from build123d import *

# Parameters (mm, degrees)
BOSS_EXTRUDE1_DEPTH = 1.2


with BuildPart() as part:
    # Sketch1 → Boss-Extrude1 (new body)
    with BuildSketch(Plane(origin=(0, 0, 0), x_dir=(1, 0, 0), z_dir=(0, 1, 0))):
        with BuildLine():
            Line((-52.420457213, 58.5), (-52.420457213, 71.946194901))
            Line((-52.420457213, 71.946194901), (-60.488236819, 80.830210159))
            Line((-60.488236819, 80.830210159), (-65.373616564, 99.749725089))
            ThreePointArc((-65.373616564, 99.749725089), (-65.730427555, 101.60979478), (-65.85, 103.5))
            Line((-65.85, 103.5), (-124.130457213, 103.5))
            Line((-124.130457213, 103.5), (-124.130457213, -71.95))
            Line((-124.130457213, -71.95), (-112.891350531, -81.0301662))
            Line((-112.891350531, -81.0301662), (-108.397048281, -103.5))
            Line((-108.397048281, -103.5), (-52.420457213, -103.5))
            Line((-52.420457213, -103.5), (-52.420457213, -58.5))
            Line((-52.420457213, -58.5), (-50.420457213, -58.5))
            Line((-50.420457213, -58.5), (-50.420457213, -145.21))
            ThreePointArc((-50.420457213, -145.21), (-48.955991119, -148.745533906), (-45.420457213, -150.21))
            Line((-45.420457213, -150.21), (42.279542787, -150.21))
            ThreePointArc((42.279542787, -150.21), (45.815076693, -148.745533906), (47.279542787, -145.21))
            Line((47.279542787, -145.21), (47.279542787, -58.5))
            Line((47.279542787, -58.5), (49.279542787, -58.5))
            Line((49.279542787, -58.5), (49.279542787, -103.5))
            Line((49.279542787, -103.5), (105.256133855, -103.5))
            Line((105.256133855, -103.5), (109.750436105, -81.0301662))
            Line((109.750436105, -81.0301662), (120.989542787, -71.95))
            Line((120.989542787, -71.95), (120.989542787, -58.5))
            Line((120.989542787, -58.5), (242.489542787, -58.5))
            Line((242.489542787, -58.5), (242.489542787, 58.5))
            Line((242.489542787, 58.5), (217.489542787, 58.5))
            Line((217.489542787, 58.5), (217.489542787, 145.21))
            ThreePointArc((217.489542787, 145.21), (216.025076693, 148.745533906), (212.489542787, 150.21))
            Line((212.489542787, 150.21), (125.989542787, 150.21))
            ThreePointArc((125.989542787, 150.21), (122.454008881, 148.745533906), (120.989542787, 145.21))
            Line((120.989542787, 145.21), (120.989542787, 58.5))
            Line((120.989542787, 58.5), (119.489542787, 58.5))
            Line((119.489542787, 58.5), (119.489542787, 103.5))
            Line((119.489542787, 103.5), (62.709085574, 103.5))
            ThreePointArc((62.709085574, 103.5), (62.589513129, 101.60979478), (62.232702138, 99.749725089))
            Line((62.232702138, 99.749725089), (57.347322393, 80.830210159))
            Line((57.347322393, 80.830210159), (49.279542787, 71.946194901))
            Line((49.279542787, 71.946194901), (49.279542787, 58.5))
            Line((49.279542787, 58.5), (8.429542787, 58.5))
            ThreePointArc((8.429542787, 58.5), (-1.570457213, 48.5), (-11.570457213, 58.5))
            Line((-11.570457213, 58.5), (-52.420457213, 58.5))
        make_face()
    extrude(amount=BOSS_EXTRUDE1_DEPTH)


solid = part.part
Build history of the part. All positions in model axes, mm. A direction names the side the tool comes from. Round coordinates to 2 decimals unless told otherwise and drop trailing zeros. Loops run counter-clockwise (first coordinate to the right, second up) from the corner with the lowest first, then second, coordinate; pieces in that order, holes last. Notation, with made-up numbers: (-15.75, 67) -> (10.25, 67) arc R32 cw to (10.25, 93) -> close; hole circle Ø5 at (82.5, 86.25). An arc over 180 degrees is marked (long way). Answer in a Markdown table with one row per item.
Item 1: Saw through at A-A (z = 96). Write the cut outline in (x, y).
Answers below:
| item | result |
|---|---|
| outline | (-109.9, 0) -> (-52.42, 0) -> (-52.42, 1.2) -> (-109.9, 1.2) -> close; (-50.42, 0) -> (47.28, 0) -> (47.28, 1.2) -> (-50.42, 1.2) -> close; (49.28, 0) -> (106.76, 0) -> (106.76, 1.2) -> (49.28, 1.2) -> close |
Item 2: Drill centre lines: L1, parallel to X at y = 0.95, z = 59.5; L2, parallel to X at y = 1.1, z = -80; L3, parallel to Z at x = 226, y = 1.1. Where is each one in solid material? Low to high. Write a range as [from, to].
Answers below:
| item | result |
|---|---|
| L1 | x = [-124.13, -52.42], [-50.42, 47.28], [49.28, 120.99] |
| L2 | x = [-124.13, -59.73], [56.59, 119.49], [120.99, 217.49] |
| L3 | z = [-58.5, 58.5] |
Item 3: Mould opens along X. For faces 1 (the flat face through (57, 0, -2)), 2 (the flat face through (-118.59, 0.592, 76.427)), 3 (the flat face through (-56.4, 0.59, -76.33)), 4 (the flat face through (115.291, 0.592, 76.554)) say: +X half, -X half, draft (parallel to the pull), parting line (faces both ways), or undercut.
Answers below:
| item | result |
|---|---|
| face 1 | draft |
| face 2 | -X half |
| face 3 | undercut |
| face 4 | +X half |
Item 4: Saw through at C-C (x = 133.5). Write the cut outline in (y, z).
Answers below:
| item | result |
|---|---|
| outline | (0, -150.21) -> (1.2, -150.21) -> (1.2, 58.5) -> (0, 58.5) -> close |
Item 5: Which spindle directions (+Z, -Z, +X, -X, +Y, -Y) get a long thin tool onto all of the face, cutting with end or side? Do faces 5 (the flat face through (53.37, 0.59, -76.45)), 6 (the flat face through (57, 1.2, -2)). Say none if no direction does.
Answers below:
| item | result |
|---|---|
| face 5 | -Z, +Y, -Y |
| face 6 | +Z, -Z, +X, -X, +Y |
Item 6: Pin check, flat tips, straight feed: pin 1 (0.6 mm diameter, centred on x = -51, y = 0.5, fed in from +Z); pin 2 (0.6 mm diameter, centred on y = 1, z = -118.5, fed in from +X); pin 3 (0.6 mm diameter, centred on y = 0.5, z = -122.5, fed in from -X). Stop position of each tip, or through.
Answers below:
| item | result |
|---|---|
| pin 1 | stops at z = 58.5 |
| pin 2 | stops at x = 217.49 |
| pin 3 | stops at x = 120.99 |
Item 7: Saw through at B-B (x = 83.5). Write the cut outline in (y, z).
Answers below:
| item | result |
|---|---|
| outline | (0, -103.5) -> (1.2, -103.5) -> (1.2, 103.5) -> (0, 103.5) -> close |
